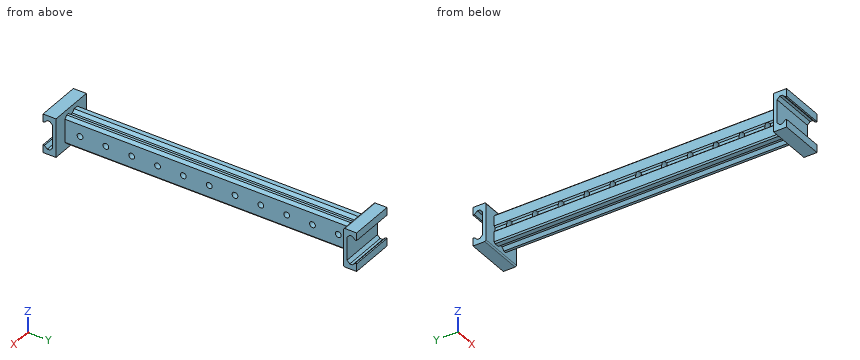
```python
from build123d import *

# Parameters (mm, degrees)
BOSS_EXTRUDE1_DEPTH = 35
FILLET1_R           = 1
BOSS_EXTRUDE2_DEPTH = 222.716603748
SKETCH6_R           = 2.238154979
CUT_EXTRUDE1_DEPTH  = 15.286677324


with BuildPart() as part:
    # Sketch1 → Boss-Extrude1 (new body)
    with BuildSketch(Plane.YZ):
        Polygon((60.116092999, 26.392150669), (61.250815122, 26.392150669), (61.250815122, 32.392150669), (51.18048308, 32.392150669), (51.18048308, 2.389198142), (61.250815122, 2.389198142), (61.250815122, 8.389198142), (60.116092999, 8.389198142), (57.992886952, 6.265992095), (55.985387253, 6.265992095), (53.862181206, 8.389198142), (53.862181206, 26.392150669), (55.985387253, 28.515356716), (57.992886952, 28.515356716), align=None)
    extrude(amount=BOSS_EXTRUDE1_DEPTH)


with BuildPart() as body_2:
    # Mirror4: mirrored copy
    add(part.part.mirror(Plane.ZX.offset(-60.177818794)))


with BuildPart() as part_1:
    add(part.part)

    # Fillet1
    fillet1_edges = [part_1.edges().sort_by_distance(p)[0] for p in [
        (17.5, 51.18048308, 2.389198142),
        (17.5, 51.18048308, 32.392150669),
    ]]
    fillet(fillet1_edges, radius=FILLET1_R)

    add(body_2.part)  # Boss-Extrude2 merges body 2
    # Sketch3 → Boss-Extrude2 (add)
    with BuildSketch(Plane.XZ.offset(-51.18048308)):
        Polygon((24.733095029, 8.333793818), (24.733095029, 26.336746345), (22.609888982, 28.459952392), (20.602389284, 28.459952392), (18.479183237, 26.336746345), (16.20973899, 26.336746345), (14.086532943, 28.459952392), (10.508020729, 28.459952392), (9.446417705, 27.398349369), (9.446417705, 19.57342506), (10.508020729, 18.511822037), (10.508020729, 16.158718126), (9.446417705, 15.097115103), (9.446417705, 7.272190794), (10.508020729, 6.210587771), (14.086532943, 6.210587771), (16.20973899, 8.333793818), (18.479183237, 8.333793818), (20.602389284, 6.210587771), (22.609888982, 6.210587771), align=None)
    extrude(amount=BOSS_EXTRUDE2_DEPTH)

    # Sketch6 → Cut-Extrude1 (cut)
    with BuildSketch(Plane(origin=(9.446417705, 0, 0), x_dir=(0, -1, 0), z_dir=(-1, 0, 0))):
        with Locations(Location((159.829006886, 17.335270082, 0), (0, 0, 90))):
            Circle(SKETCH6_R)
        with Locations(Location((139.829006886, 17.335270082, 0), (0, 0, 90))):
            Circle(SKETCH6_R)
        with Locations(Location((119.829006886, 17.335270082, 0), (0, 0, 90))):
            Circle(SKETCH6_R)
        with Locations(Location((99.829006886, 17.335270082, 0), (0, 0, 90))):
            Circle(SKETCH6_R)
        with Locations(Location((79.829006886, 17.335270082, 0), (0, 0, 90))):
            Circle(SKETCH6_R)
        with Locations(Location((59.829006886, 17.335270082, 0), (0, 0, 90))):
            Circle(SKETCH6_R)
        with Locations(Location((39.829006886, 17.335270082, 0), (0, 0, 90))):
            Circle(SKETCH6_R)
        with Locations(Location((19.829006886, 17.335270082, 0), (0, 0, 90))):
            Circle(SKETCH6_R)
        with Locations(Location((-0.170993114, 17.335270082, 0), (0, 0, 90))):
            Circle(SKETCH6_R)
        with Locations(Location((-20.170993114, 17.335270082, 0), (0, 0, 90))):
            Circle(SKETCH6_R)
        with Locations(Location((-40.170993114, 17.335270082, 0), (0, 0, 90))):
            Circle(SKETCH6_R)
    extrude(amount=-CUT_EXTRUDE1_DEPTH, mode=Mode.SUBTRACT)


solid = part_1.part
```
For this review, take the finished solid that the model builds, in its own axes (mm). Round coordinates to 2 decimals unless told otherwise and drop trailing zeros. Write each loop counter-clockwise with the first axis right and the second up, starting at its lowest first coordinate (ties: lowest second). Pieces come first, ordered by that corner, then holes. Notation, with made-up numbers: M 16.5,82.25 L 61.5,82.25 A14 cw 61.5,90.25 Z; hole C 70.5,55.25 d3. An arc over 180 degrees is marked long. One line per item, written item: value. Start each with the question number.
(1) We need section A-A (y = -11). Give the boundary of the cut face in (x, z).
(2) We need section B-B (z = 23). Give the boundary of the cut face in (x, y), and give its area (3 significant figures).
(3) Insertion check: pin 1 (7 mm diameter, centred on y = -19.83, z = 17.34, fed in from -X); pin 2 (2 mm diameter, centred on y = -73.5, z = 15.5, fed in from +X); pin 3 (1.9 mm diameter, centred on y = -129.5, z = 17.5, fed in from -X). Each pin has a flat end and moves straight along its axis. Give the tip position at first contact, or say it passes through.
(4) Wall thickness on line 1 (Y direction, x = 8, z = 4); line 2 (Y direction, x = 30, z = 24); line 3 (Y direction, x = 2, z = 27): over which ranges is each line inside the solid? List them lowest first.
Result:
1. outline: M 9.45,7.27 L 10.51,6.21 L 14.09,6.21 L 16.21,8.33 L 18.48,8.33 L 20.6,6.21 L 22.61,6.21 L 24.73,8.33 L 24.73,26.34 L 22.61,28.46 L 20.6,28.46 L 18.48,26.34 L 16.21,26.34 L 14.09,28.46 L 10.51,28.46 L 9.45,27.4 L 9.45,19.57 L 10.51,18.51 L 10.51,16.16 L 9.45,15.1 Z
2. outline: M 0,-174.22 L 35,-174.22 L 35,-171.54 L 24.73,-171.54 L 24.73,51.18 L 35,51.18 L 35,53.86 L 0,53.86 L 0,51.18 L 9.45,51.18 L 9.45,-171.54 L 0,-171.54 Z
2. area: 3,590 mm²
3. pin 1: x = 9.45
3. pin 2: x = 24.73
3. pin 3: x = 10.51
4. line 1: -181.61 to -171.54, 51.18 to 61.25
4. line 2: -174.22 to -171.54, 51.18 to 53.86
4. line 3: -181.61 to -179.86, -174.83 to -171.54, 51.18 to 54.47, 59.51 to 61.25
